Verification items for this drawing (mm, ordinates from the low corner). Give positions to 0.01 mm unless a question says otherwise; leave off trailing zeros. Loops run counter-clockwise (first coordinate to the right, second up) from the corner with the lowest first, then second, coordinate; pieces in that order, holes last. Notation, with made-up numbers: (45, -24.75) - (61, -24.75) arc R24 ccw to (61, 5.25) - close; hole circle Ø10 at (89.5, 68). An arc over 180 degrees is marked (long way). Write item = value, one per line. Start each with the question number.
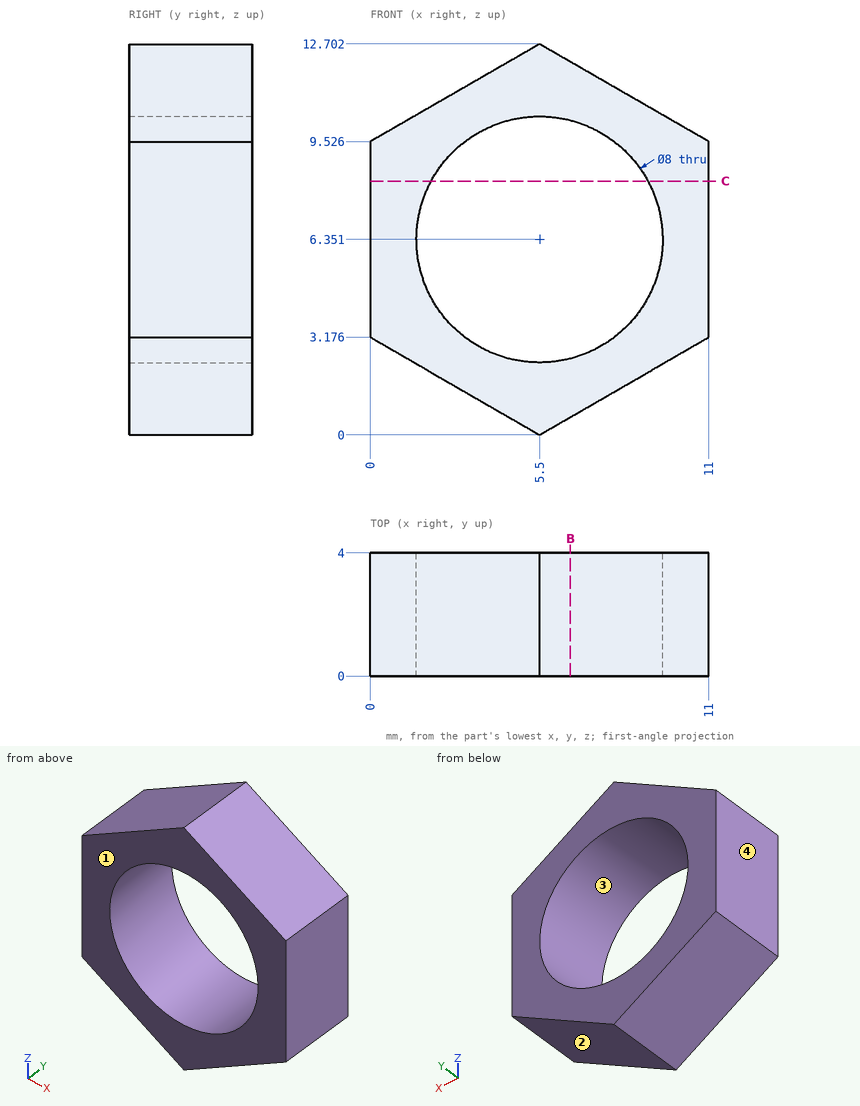
1) Cross-section at C-C on z = 8.25. Enter the section's corners in (x, y).
2) Cross-section at B-B on x = 6.5. Enter the section's corners in (y, z) (1 decimal).
3) Material ranges on line 1 along X through (y, z) = (1.45, 8) (1 decimal); line 2 along X through (y, z) = (2.7, 4) (1 decimal); line 3 along Z through (x, y) = (7.5, 2.65) (1 decimal), recorded low to high.
4) Release check for a two-part mould opening along X. For the marked faces 1, 2, 3 and 4 record: pulls with the +X half, pulls with the -X half, needs draft (parallel to the pull), parting line crosses it, or undercut.
Checked values:
q1.outline = (0, 0) - (1.98, 0) - (1.98, 4) - (0, 4) - close; (9.02, 0) - (11, 0) - (11, 4) - (9.02, 4) - close
q2.outline = (0, 0.6) - (4, 0.6) - (4, 2.5) - (0, 2.5) - close; (0, 10.2) - (4, 10.2) - (4, 12.1) - (0, 12.1) - close
q3.line_1 = 0 to 1.9, 9.1 to 11
q3.line_2 = 0 to 2.3, 8.7 to 11
q3.line_3 = 1.2 to 2.9, 9.8 to 11.5
q4.face_1 = needs draft
q4.face_2 = pulls with the +X half
q4.face_3 = undercut
q4.face_4 = pulls with the -X half
